Check sheet for the modelled part. Datum: model origin and axes. Units: mm. Face numbers are marked on the shaded views. A direction names the side the tool comes from. Give positions to 0.01 mm unless a question says otherwise; leave off trailing zeros. Write each loop counter-clockwise with the first axis right and the second up, starting at its lowest first coordinate (ties: lowest second). Pieces come first, ordered by that corner, then holes. Notation, with made-up numbers: (-22, -30.5) -> (-4, -30.5) arc R23 cw to (-4, -18.5) -> close; hole circle Ø6 at (72.25, 23). An arc over 180 degrees is marked (long way). Use a Markdown table: item, result. Add a question column.
1. Cross-section at D-D (z = 18). Enter the section's corners in (x, y), then the cut area to 3 significant figures.
2. Cross-section at A-A (y = 0). Enter the section's corners in (x, z).
3. Cross-section at B-B (z = 10). Enter the section's corners in (x, y), then the cut area to 3 significant figures.
4. Scan lines: probe 1 along Y at (x, z) = (2.6, 10); probe 2 along Y at (x, z) = (2.1, -0.5); probe 3 along Z at (x, y) = (4.85, 2). Record each from-to range of solid material in increasing order. Write a range as [from, to].
5. Set-up check for the marked faces 1, 2 and 3: record each of +Z, -Z, +X, -X, +Y, -Y from which the full face is reachable in a straight line by a thin tool's end or side.
6. Gauge pin test, flat ends, axial feed: P1, Ø2, axis at x = 4.5, z = 13, coming from the +Y side; P2, Ø2.5, axis at x = 2, y = 17, coming from the -Z side; P3, Ø0.9, axis at x = 3, y = 16, coming from the +Z side; P4, Ø6, axis at y = -2.5, z = -12.5, coming from the -X side. Record the tip position at first contact, or that the pin passes through.
7. Cross-section at C-C (x = 2.5). Enter the section's corners in (y, z).
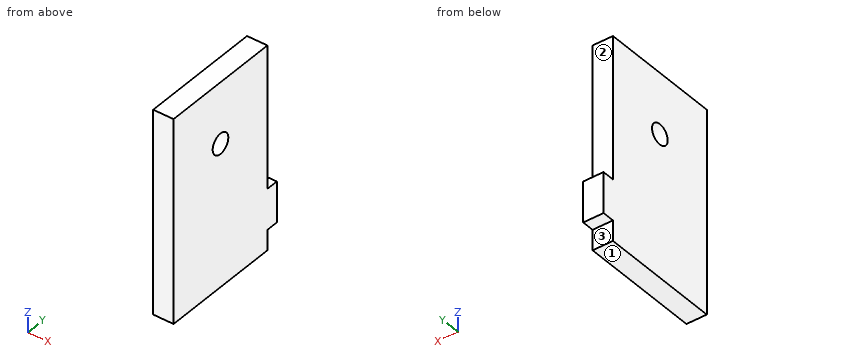
from build123d import *

# Parameters (mm, degrees)
SKETCH1_W          = 50
SKETCH1_H          = 30
EXTRUDE1_DEPTH     = 5
SKETCH2_W          = 10
SKETCH2_H          = 3
EXTRUDE2_DEPTH     = 5
SKETCH3_R          = 2.5
CUT_EXTRUDE1_DEPTH = 32.208973069


with BuildPart() as part:
    # Sketch1 → Extrude1 (new body)
    with BuildSketch(Plane(origin=(0, 0, 0), x_dir=(0, 0, -1), z_dir=(1, 0, 0))):
        Rectangle(SKETCH1_W, SKETCH1_H)
    extrude(amount=EXTRUDE1_DEPTH)

    # Sketch2 → Extrude2 (add)
    with BuildSketch(Plane(origin=(5, 0, 0), x_dir=(0, 0, -1), z_dir=(1, 0, 0))):
        with Locations((15, 16.5)):
            Rectangle(SKETCH2_W, SKETCH2_H)
    extrude(amount=-EXTRUDE2_DEPTH)

    # Sketch3 → Cut-Extrude1 (cut, through all)
    with BuildSketch(Plane(origin=(5, 0, 0), x_dir=(0, 0, -1), z_dir=(1, 0, 0))):
        with Locations((-10, 0)):
            Circle(SKETCH3_R)
    extrude(amount=-CUT_EXTRUDE1_DEPTH, mode=Mode.SUBTRACT)


solid = part.part
Worked answers:
| question | item | result |
|---|---|---|
| 1 | outline | (0, -15) -> (5, -15) -> (5, 15) -> (0, 15) -> close |
| 1 | area | 150 mm² |
| 2 | outline | (0, -25) -> (5, -25) -> (5, 7.5) -> (0, 7.5) -> close; (0, 12.5) -> (5, 12.5) -> (5, 25) -> (0, 25) -> close |
| 3 | outline | (0, -15) -> (5, -15) -> (5, -2.5) -> (0, -2.5) -> close; (0, 2.5) -> (5, 2.5) -> (5, 15) -> (0, 15) -> close |
| 3 | area | 125 mm² |
| 4 | probe 1 | y = [-15, -2.5], [2.5, 15] |
| 4 | probe 2 | y = [-15, 15] |
| 4 | probe 3 | z = [-25, 8.5], [11.5, 25] |
| 5 | face 1 | -Z, +X, -X, +Y, -Y |
| 5 | face 2 | +Z, +X, -X, +Y |
| 5 | face 3 | -Z, +X, -X, +Y |
| 6 | P1 | stops at y = 15 |
| 6 | P2 | stops at z = -20 |
| 6 | P3 | stops at z = -10 |
| 6 | P4 | stops at x = 0 |
| 7 | outline | (-15, -25) -> (15, -25) -> (15, -20) -> (18, -20) -> (18, -10) -> (15, -10) -> (15, 25) -> (-15, 25) -> close; hole circle Ø5 at (0, 10) |
